The listing builds one solid part. Answer for the finished solid, in the listing's coordinates (mm). Give positions to 0.01 mm unless a question says otherwise; leave off trailing zeros. Order: outer loops, then holes, each group sorted by start corner. A loop starts at its lowest first (then second) coordinate and runs counter-clockwise, first axis right, second up. Notation, with made-up numbers: (36, 86) - (45, 86) arc R15 ccw to (45, 105) - close; hole circle Ø4 at (49, 82). An arc over 180 degrees is marked (long way). Answer as a JSON object with one key per item and string values. Group by question number.
Q1. A cutting plane is placed at A-A, the plane z = 2.55. Count the separate pieces of the cut face and the enclosed holes in it, and give its area (3 significant figures).
Q2. A cutting plane is placed at C-C, the plane x = 13.45. Give the vertices of the cut face in (y, z), and give its area (3 significant figures).
Q3. Given pin 1 (0.6 mm diameter, centred on x = 15, z = 3.5, fed in from +Y), flat-ended and moving along its own axis, determine where the tip first touches the part or whether it passes through.
Q4. Consider line 1 (Y direction, x = 13.5, z = 2.15); line 2 (X direction, y = 30.71, z = 3.15); line 3 (Y direction, x = 6, z = 3.5). Determine where each line is inside the solid, lowest interval first.
Q5. A cutting plane is placed at D-D, the plane x = 10.2. Give the vertices of the cut face in (y, z).
Q6. A cutting plane is placed at B-B, the plane y = 9.5. Give the vertices of the cut face in (x, z).
from build123d import *

# Parameters (mm, degrees)
SKETCH1_R           = 0.85
BOSS_EXTRUDE1_DEPTH = 4
SKETCH2_W           = 16.2
SKETCH2_H           = 33.21
CUT_EXTRUDE2_DEPTH  = 2


with BuildPart() as part:
    # Sketch1 → Boss-Extrude1 (new body)
    with BuildSketch(Plane.XY):
        with BuildLine():
            Line((0, 26.21), (0, 7))
            Line((0, 7), (4, 7))
            Line((4, 7), (4, 5))
            Line((4, 5), (0, 5))
            Line((0, 5), (0, 2))
            ThreePointArc((0, 2), (0.585786438, 0.585786438), (2, 0))
            Line((2, 0), (14.2, 0))
            ThreePointArc((14.2, 0), (15.614213562, 0.585786438), (16.2, 2))
            Line((16.2, 2), (16.2, 5))
            Line((16.2, 5), (12.2, 5))
            Line((12.2, 5), (12.2, 7))
            Line((12.2, 7), (16.2, 7))
            Line((16.2, 7), (16.2, 26.21))
            Line((16.2, 26.21), (12.2, 26.21))
            Line((12.2, 26.21), (12.2, 28.21))
            Line((12.2, 28.21), (16.2, 28.21))
            Line((16.2, 28.21), (16.2, 31.21))
            ThreePointArc((16.2, 31.21), (15.614213562, 32.624213562), (14.2, 33.21))
            Line((14.2, 33.21), (2, 33.21))
            ThreePointArc((2, 33.21), (0.585786438, 32.624213562), (0, 31.21))
            Line((0, 31.21), (0, 28.21))
            Line((0, 28.21), (4, 28.21))
            Line((4, 28.21), (4, 26.21))
            Line((4, 26.21), (0, 26.21))
        make_face()
        with Locations((13.45, 2.5)):
            Circle(SKETCH1_R, mode=Mode.SUBTRACT)
        with Locations((10.2, 9.5)):
            Circle(SKETCH1_R, mode=Mode.SUBTRACT)
        with Locations((2.75, 30.71)):
            Circle(SKETCH1_R, mode=Mode.SUBTRACT)
        with Locations((6, 23.71)):
            Circle(SKETCH1_R, mode=Mode.SUBTRACT)
        with Locations((6, 9.5)):
            Circle(SKETCH1_R, mode=Mode.SUBTRACT)
        with Locations((2.75, 2.5)):
            Circle(SKETCH1_R, mode=Mode.SUBTRACT)
        with Locations((10.2, 23.71)):
            Circle(SKETCH1_R, mode=Mode.SUBTRACT)
        with Locations((13.45, 30.71)):
            Circle(SKETCH1_R, mode=Mode.SUBTRACT)
    extrude(amount=BOSS_EXTRUDE1_DEPTH)

    # Sketch2 → Cut-Extrude2 (cut)
    with BuildSketch(Plane.XY):
        with Locations((8.1, 16.605)):
            Rectangle(SKETCH2_W, SKETCH2_H)
    extrude(amount=CUT_EXTRUDE2_DEPTH, mode=Mode.SUBTRACT)


solid = part.part
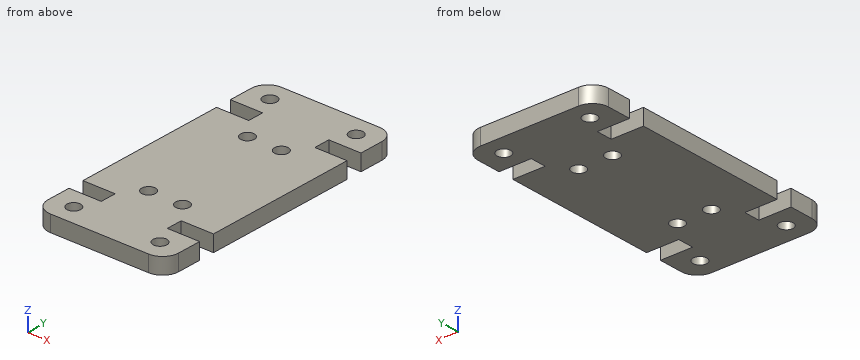
Reply:
{
 "1": {"separate pieces": "1", "enclosed holes": "8", "area": "484 mm^2"},
 "2": {"outline": "(0, 2) - (1.65, 2) - (1.65, 4) - (0, 4) - close; (3.35, 2) - (5, 2) - (5, 4) - (3.35, 4) - close; (7, 2) - (26.21, 2) - (26.21, 4) - (7, 4) - close; (28.21, 2) - (29.86, 2) - (29.86, 4) - (28.21, 4) - close; (31.56, 2) - (33.21, 2) - (33.21, 4) - (31.56, 4) - close", "area": "51.6 mm^2"},
 "3": {"pin 1": "stops at y = 33.15"},
 "4": {"line 1": "y = 0 to 1.65, 3.35 to 5, 7 to 26.21, 28.21 to 29.86, 31.56 to 33.21", "line 2": "x = 0 to 1.9, 3.6 to 12.6, 14.3 to 16.2", "line 3": "y = 0 to 8.65, 10.35 to 22.86, 24.56 to 33.21"},
 "5": {"outline": "(0, 2) - (8.65, 2) - (8.65, 4) - (0, 4) - close; (10.35, 2) - (22.86, 2) - (22.86, 4) - (10.35, 4) - close; (24.56, 2) - (33.21, 2) - (33.21, 4) - (24.56, 4) - close"},
 "6": {"outline": "(0, 2) - (5.15, 2) - (5.15, 4) - (0, 4) - close; (6.85, 2) - (9.35, 2) - (9.35, 4) - (6.85, 4) - close; (11.05, 2) - (16.2, 2) - (16.2, 4) - (11.05, 4) - close"}
}
